```python
from build123d import *

# Parameters (mm, degrees)
F0_W     = 87.960623
F0_H     = 58.109455
F1_DEPTH = 127
F3_DEPTH = 129.286
F5_DEPTH = 123.952


with BuildPart() as f1:
    # F0 (on Front) → F1 (new body)
    with BuildSketch(Plane.XZ):
        with Locations((-0.927712, 2.336059)):
            Rectangle(F0_W, F0_H)
    extrude(amount=F1_DEPTH)

    # F2 (on face) → F3 (join)
    with BuildSketch(Plane.XZ.offset(127)):
        Polygon((0, 66.431664), (-44.908024, 31.390786), (43.052599, 31.390786), align=None)
    extrude(amount=-F3_DEPTH)

    # F4 (on face) → F5 (join)
    with BuildSketch(Plane.XZ.offset(127)):
        Polygon((76.651916, 31.390786), (43.052599, 31.390786), (43.052599, -26.718669), (76.651916, -27.594689), align=None)
    extrude(amount=-F5_DEPTH)


solid = f1.part
```
Read the model definition and answer for the solid it produces. Units are mm, in the model's axes. A direction names the side the tool comes from. Give positions to 0.01 mm unless a question says otherwise; leave off trailing zeros. Write each loop counter-clockwise with the first axis right and the second up, starting at its lowest first coordinate (ties: lowest second). Pieces come first, ordered by that corner, then holes. Notation, with made-up numbers: (8, 43) -> (28, 43) arc R11 cw to (28, 58) -> close; hole circle Ø9 at (-26.75, 80.25). An arc over 180 degrees is marked (long way). Answer in a Markdown table with one row per item.
1) Section C-C on x = 4.5 is taken. Give the vertices of the cut face in (y, z).
Results list:
| item | result |
|---|---|
| outline | (-127, -26.72) -> (0, -26.72) -> (0, 31.39) -> (2.29, 31.39) -> (2.29, 62.77) -> (-127, 62.77) -> close |
2) Section D-D on z = 35.5 is taken. Give the vertices of the cut face in (x, y), plus the area to 3 significant figures.
Results list:
| item | result |
|---|---|
| outline | (-39.64, -127) -> (38, -127) -> (38, 2.29) -> (-39.64, 2.29) -> close |
| area | 10,000 mm^2 |
3) A tool of negligible diameter and unlimited length cuts with its end or side. For faces 1 (the flat face through (43.053, -2, 2)), 2 (the flat face through (-2, -63, -26.719)), 3 (the flat face through (60, -66, 31.391)), 4 (the flat face through (-2, 0, 3)), from which of +Z, -Z, +X, -X, +Y, -Y can it reach the whole face along a straight path? Write none if from no direction.
Results list:
| item | result |
|---|---|
| face 1 | +Z, -Z, +X, +Y |
| face 2 | -Z, -X, +Y, -Y |
| face 3 | +Z, +X, +Y, -Y |
| face 4 | -Z, +X, -X, +Y |
4) Straight lines are drawn through the part: line 1 (Y direction, x = 31.5, z = 8); line 2 (Y direction, x = 54, z = -20.5); line 3 (X direction, y = -74.5, z = 35). For each, find the intervals that lie inside material, in ascending order. Write a range as [from, to].
Results list:
| item | result |
|---|---|
| line 1 | [-127, 0] |
| line 2 | [-127, -3.05] |
| line 3 | [-40.28, 38.62] |
5) Section B-B on y = -95 is taken. Give the vertices of the cut face in (x, z).
Results list:
| item | result |
|---|---|
| outline | (-44.91, -26.72) -> (43.05, -26.72) -> (76.65, -27.59) -> (76.65, 31.39) -> (43.05, 31.39) -> (0, 66.43) -> (-44.91, 31.39) -> close |
6) Section A-A on z = -17.5 is taken. Give the vertices of the cut face in (x, y), plus the area to 3 significant figures.
Results list:
| item | result |
|---|---|
| outline | (-44.91, -127) -> (76.65, -127) -> (76.65, -3.05) -> (43.05, -3.05) -> (43.05, 0) -> (-44.91, 0) -> close |
| area | 15,300 mm^2 |
7) Each of these flat-tipped pins is pushed along its axis until it touches: pin 1 Ø1 at (x, y) = (-11, -65.5) entering from +Z; pin 2 Ø1 at (y, z) = (-73, 42.5) entering from -X; pin 3 Ø2 at (x, z) = (-11, 25.5) entering from +Y. Where does it stop, or does it pass through?
Results list:
| item | result |
|---|---|
| pin 1 | z = 58.24 |
| pin 2 | x = -31.31 |
| pin 3 | y = 0 |
